from build123d import *

# Parameters (mm, degrees)
ESQUISSE1_R                                        = 12
BOSS_EXTRU_1_DEPTH                                 = 3.91
ESQUISSE6_R                                        = 4
ENL_V_MAT_EXTRU_2_DEPTH                            = 1.91
ESQUISSE7_R                                        = 4.95
ESQUISSE7_R_2                                      = 3.25
BOSS_EXTRU_2_DEPTH                                 = 9.75
CHAMBRAGE_POUR_VIS_T_TE_RONDE_BOMB_E_M_D           = 2.4
CHAMBRAGE_POUR_VIS_T_TE_RONDE_BOMB_E_M_CBORE_D     = 5
CHAMBRAGE_POUR_VIS_T_TE_RONDE_BOMB_E_M_CBORE_DEPTH = 1.6
R_P_TITION_CIRCULAIRE2_COUNT                       = 4
ENL_V_MAT_EXTRU_3_DEPTH                            = 22.78521517
ENL_V_MAT_EXTRU_3_DEPTH_BACK                       = 22.78521517
ESQUISSE12_R                                       = 1.45


with BuildPart() as part:
    # Esquisse1 → Boss.-Extru.1 (new body)
    with BuildSketch(Plane.XY):
        Circle(ESQUISSE1_R)
    extrude(amount=BOSS_EXTRU_1_DEPTH)

    # Esquisse6 → Enlèv. mat.-Extru.2 (cut)
    with BuildSketch(Plane(origin=(0, 0, 0), x_dir=(-1, 0, 0), z_dir=(0, 0, -1))):
        Circle(ESQUISSE6_R)
    extrude(amount=-ENL_V_MAT_EXTRU_2_DEPTH, mode=Mode.SUBTRACT)

    # Esquisse7 → Boss.-Extru.2 (add)
    with BuildSketch(Plane.XY.offset(3.91)):
        Circle(ESQUISSE7_R)
        Circle(ESQUISSE7_R_2, mode=Mode.SUBTRACT)
    extrude(amount=BOSS_EXTRU_2_DEPTH)

    # Chambrage pour vis à tête ronde bombée M21 (through all)
    with Locations(Plane.XY.offset(3.91)):
        with Locations((0, 8)):
            chambrage_pour_vis_t_te_ronde_bomb_e_m = CounterBoreHole(CHAMBRAGE_POUR_VIS_T_TE_RONDE_BOMB_E_M_D / 2, CHAMBRAGE_POUR_VIS_T_TE_RONDE_BOMB_E_M_CBORE_D / 2, CHAMBRAGE_POUR_VIS_T_TE_RONDE_BOMB_E_M_CBORE_DEPTH)

    # Répétition circulaire2: Chambrage pour vis à tête ronde bombée M21 ×4 about axis
    r_p_tition_circulaire2_axis = Axis((0, 0, 0), (0, 0, 1))
    for i in range(1, R_P_TITION_CIRCULAIRE2_COUNT):
        add(chambrage_pour_vis_t_te_ronde_bomb_e_m.rotate(r_p_tition_circulaire2_axis, i * 360 / R_P_TITION_CIRCULAIRE2_COUNT), mode=Mode.SUBTRACT)

    # Esquisse12 → Enlèv. mat.-Extru.3 (cut, two sides: drawn at the far end of the back side and taken through both)
    with BuildSketch(Plane(origin=(0, 0, 0), x_dir=(1, 0, 0), z_dir=(0, 1, 0)).offset(-ENL_V_MAT_EXTRU_3_DEPTH_BACK)):
        with Locations(Location((0, -8.785, 0), (0, 0, 270))):
            Circle(ESQUISSE12_R)
    extrude(amount=ENL_V_MAT_EXTRU_3_DEPTH + ENL_V_MAT_EXTRU_3_DEPTH_BACK, mode=Mode.SUBTRACT)


solid = part.part
The model under review builds one solid part; all positions refer to its coordinate system, in mm. A direction names the side the tool comes from. Give positions to 0.01 mm unless a question says otherwise; leave off trailing zeros. Loops run counter-clockwise (first coordinate to the right, second up) from the corner with the lowest first, then second, coordinate; pieces in that order, holes last. Notation, with made-up numbers: (55, 59) -> (70, 59) arc R17 cw to (70, 68) -> close; hole circle Ø7 at (-2, 82). An arc over 180 degrees is marked (long way). Write each question's results on one line, items separated by ' | '.
1) Tool access review of faces 1 (the face through (3.1, 0.98, 8.72)), 2 (the face through (0, 0, 1.91)), 3 (the face through (-9.01, -0.65, 1.14)): name each direction out of +Z, -Z, +X, -X, +Y, -Y from which nothing blocks a thin tool from reaching the whole face with its end or side.
Conclusion:
face 1: +Z | face 2: -Z | face 3: +Z, -Z
2) Take a section at B-B, the plane y = -8. Give the boundary of the cut face in (x, z).
Conclusion:
outline: (-8.94, 0) -> (-1.2, 0) -> (-1.2, 2.31) -> (-2.5, 2.31) -> (-2.5, 3.91) -> (-8.94, 3.91) -> close; (1.2, 0) -> (8.94, 0) -> (8.94, 3.91) -> (2.5, 3.91) -> (2.5, 2.31) -> (1.2, 2.31) -> close
3) Insertion check: pin 1 Ø2.5 at (x, y) = (-1, 0) entering from -Z; pin 2 Ø1.4 at (x, y) = (8, 0) entering from -Z; pin 3 Ø5 at (y, z) = (-4.5, 8) entering from +X; pin 4 Ø2.5 at (x, y) = (-7.5, -1) entering from +Z. Each pin has a flat end and moves straight along its axis. Give the tip position at first contact, or say it passes through.
Conclusion:
pin 1: stops at z = 1.91 | pin 2: passes through | pin 3: stops at x = 4.53 | pin 4: stops at z = 2.31
4) Take a section at A-A, the plane y = 0. Count the separate pieces of the cut face and the enclosed holes in it, plus the area to 3 significant figures.
Conclusion:
separate pieces: 3 | enclosed holes: 0 | area: 84.6 mm^2
5) Draft analysis for pull direction Y (two halves, no side actions). For faces 4 (the face through (9.01, 0.65, 1.14)), 5 (the face through (2.284, -4.392, 8.717)), 6 (the face through (5.2, 0.2, 3.91)), state which applies: pulls with the +Y half, pulls with the -Y half, needs draft (parallel to the pull), parting line crosses it, or undercut.
Conclusion:
face 4: undercut | face 5: parting line crosses it | face 6: needs draft
6) For line 1 along Y through (x, z) = (0, 2.85); line 2 along Y through (x, z) = (0, 0.6); line 3 along Z through (x, y) = (0, 3.7) (3 decimals), list the stretches that pass through material, from the lowest coordinate up. Write a range as from..to.
Conclusion:
line 1: y = -12..-10.5, -5.5..5.5, 10.5..12 | line 2: y = -12..-9.2, -6.8..-4, 4..6.8, 9.2..12 | line 3: z = 1.91..7.335, 10.235..13.66
7) Take a section at D-D, the plane z = 5.5. Give the boundary of the cut face in (x, y), plus the area to 3 significant figures.
Conclusion:
outline: circle Ø9.9 at (0, 0); hole circle Ø6.5 at (0, 0) | area: 43.8 mm^2
